Read the model definition and answer for the solid it produces. Units are mm, in the model's axes. Give positions to 0.01 mm unless a question says otherwise; leave off trailing zeros. Write each loop counter-clockwise with the first axis right and the second up, starting at its lowest first coordinate (ties: lowest second). Pieces come first, ordered by that corner, then holes.
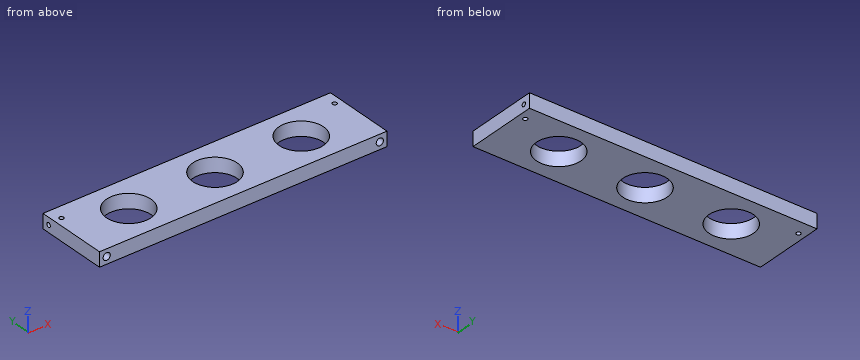
```python
from build123d import *

# Parameters (mm, degrees)
SKETCH1_W           = 200
SKETCH1_H           = 50
SKETCH1_R           = 15.5
SKETCH1_R_2         = 1.5
BOSS_EXTRUDE1_DEPTH = 10
SKETCH2_R           = 2.5
CUT_EXTRUDE1_DEPTH  = 10
SKETCH3_R           = 1.5
CUT_EXTRUDE2_DEPTH  = 200


with BuildPart() as part:
    # Sketch1 → Boss-Extrude1 (new body)
    with BuildSketch(Plane.XY):
        Rectangle(SKETCH1_W, SKETCH1_H)
        Circle(SKETCH1_R, mode=Mode.SUBTRACT)
        with Locations((60, 0)):
            Circle(SKETCH1_R, mode=Mode.SUBTRACT)
        with Locations((-60, 0)):
            Circle(SKETCH1_R, mode=Mode.SUBTRACT)
        with Locations((95, 15)):
            Circle(SKETCH1_R_2, mode=Mode.SUBTRACT)
        with Locations((-95, 15)):
            Circle(SKETCH1_R_2, mode=Mode.SUBTRACT)
    extrude(amount=BOSS_EXTRUDE1_DEPTH)

    # Sketch2 → Cut-Extrude1 (cut)
    with BuildSketch(Plane.XZ.offset(25)):
        with Locations(Location((-95, 5, 0), (0, 0, 270))):
            Circle(SKETCH2_R)
        with Locations(Location((95, 5, 0), (0, 0, 270))):
            Circle(SKETCH2_R)
    extrude(amount=-CUT_EXTRUDE1_DEPTH, mode=Mode.SUBTRACT)

    # Sketch3 → Cut-Extrude2 (cut)
    with BuildSketch(Plane(origin=(100, 0, 0), x_dir=(0, 0, -1), z_dir=(1, 0, 0))):
        with Locations((-5, 20)):
            Circle(SKETCH3_R)
    extrude(amount=-CUT_EXTRUDE2_DEPTH, mode=Mode.SUBTRACT)


solid = part.part
```
Item 1: Find the intervals of material crossed by line 1 along Y through (x, z) = (-66, 6); line 2 along Y through (x, z) = (60, 2); line 3 along X through (y, z) = (6.5, 1.5), in increasing order.
Result set:
line 1: y = -25 to -14.29, 14.29 to 18.88, 21.12 to 25
line 2: y = -25 to -15.5, 15.5 to 25
line 3: x = -100 to -74.07, -45.93 to -14.07, 14.07 to 45.93, 74.07 to 100
Item 2: Section D-D (x = -52.5) is taken. Write down the section's boundary in (y, z).
Result set:
outline: (-25, 0) - (-13.56, 0) - (-13.56, 10) - (-25, 10) - close; (13.56, 0) - (25, 0) - (25, 10) - (13.56, 10) - close; hole circle Ø3 at (20, 5)
Item 3: Section C-C (y = 0) is taken. Write down the section's boundary in (x, z), and give its area (3 significant figures).
Result set:
outline: (-100, 0) - (-75.5, 0) - (-75.5, 10) - (-100, 10) - close; (-44.5, 0) - (-15.5, 0) - (-15.5, 10) - (-44.5, 10) - close; (15.5, 0) - (44.5, 0) - (44.5, 10) - (15.5, 10) - close; (75.5, 0) - (100, 0) - (100, 10) - (75.5, 10) - close
area: 1,070 mm2
Item 4: Section B-B (x = 0) is taken. Write down the section's boundary in (y, z).
Result set:
outline: (-25, 0) - (-15.5, 0) - (-15.5, 10) - (-25, 10) - close; (15.5, 0) - (25, 0) - (25, 10) - (15.5, 10) - close; hole circle Ø3 at (20, 5)
Item 5: Section A-A (z = 5) is taken. Write down the section's boundary in (x, y).
Result set:
outline: (-100, -25) - (-97.5, -25) - (-97.5, -15) - (-92.5, -15) - (-92.5, -25) - (92.5, -25) - (92.5, -15) - (97.5, -15) - (97.5, -25) - (100, -25) - (100, 18.5) - (-100, 18.5) - close; (-100, 21.5) - (100, 21.5) - (100, 25) - (-100, 25) - close; hole circle Ø3 at (-95, 15); hole circle Ø31 at (-60, 0); hole circle Ø31 at (0, 0); hole circle Ø31 at (60, 0); hole circle Ø3 at (95, 15)
